Source: three-view drawing plus pictorial views. Frame: mm from the lowest corner of the part. A direction names the side the tool comes from. Give positions to 0.01 mm unless a question says otherwise; leave off trailing zeros. Order: outer loops, then holes, each group sorted by start corner. A loop starts at its lowest first (then second) coordinate and runs counter-clockwise, first axis right, second up. Notation, with made-up numbers: M -10,26.25 L 44,26.25 A17 ccw 44,42.25 Z; hole C 81.5,-26 d9. An arc over 180 degrees is marked long. One line per item, written item: value. Start each with the question number.
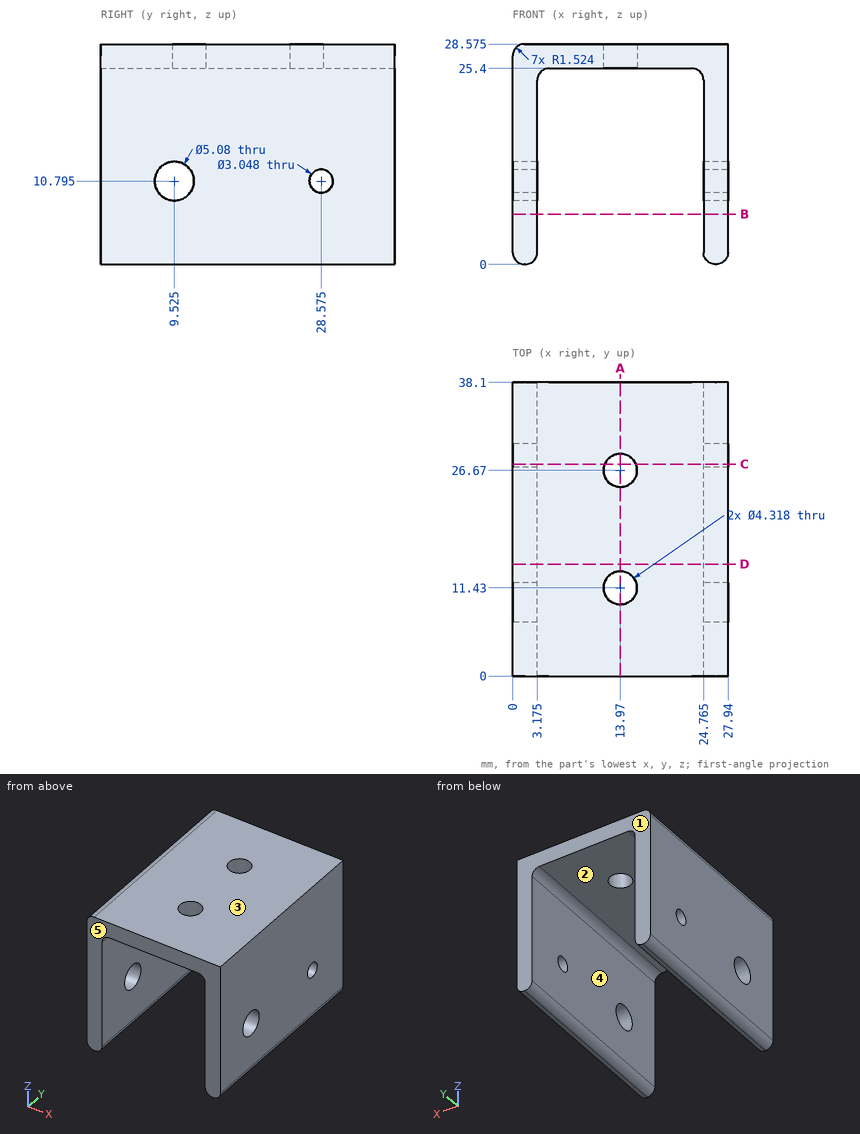
Q1. Mould query, pull axis Z, two halves, no side actions, for the marked faces 1, 2 and 3. Classes: +Z half, -Z half, draft (parallel to the pull), parting line (faces both ways), or undercut.
Q2. Section query A-A on x = 13.97. Return loops of the section in (y, z) (3 decimals), and give its area (3 significant figures).
Q3. Contact query for a flat-ended pin moving along its axis: pin 1 (3.5 mm diameter, centred on x = 13.97, y = 11.43, fed in from -Z). Output: stop coordinate, or through.
Q4. Section query B-B on z = 6.5. Return loops of the section in (x, y) (3 decimals).
Q5. Section query D-D on y = 14.5. Return loops of the section in (x, z) (3 decimals).
Q6. Section query C-C on y = 27.5. Return loops of the section in (x, z) (3 decimals), and give its area (3 significant figures).
Q7. Set-up query: the marked faces 4 and 5. Return all of +Z, -Z, +X, -X, +Y, -Y with unobstructed straight access to the full face (end or side cutting, diameter ignored); none if empty.
Q8. Ray query, line 1 along Y through (x, z) = (13.97, 27.5); line 2 along X through (y, z) = (23.5, 19.5) (3 decimals); line 3 along Y through (x, z) = (26, 9.5). Return the intervals inside material, ascending. Write a range as [from, to].
Results below:
1. face 1: draft
1. face 2: -Z half
1. face 3: +Z half
2. outline: M 0,25.4 L 9.271,25.4 L 9.271,28.575 L 0,28.575 Z; M 13.589,25.4 L 24.511,25.4 L 24.511,28.575 L 13.589,28.575 Z; M 28.829,25.4 L 38.1,25.4 L 38.1,28.575 L 28.829,28.575 Z
2. area: 93.5 mm2
3. pin 1: through
4. outline: M 0,0 L 3.175,0 L 3.175,38.1 L 0,38.1 Z; M 24.765,0 L 27.94,0 L 27.94,38.1 L 24.765,38.1 Z
5. outline: M 0,1.524 A1.524 ccw 1.524,0 L 1.651,0 A1.524 ccw 3.175,1.524 L 3.175,23.876 A1.524 cw 4.699,25.4 L 23.241,25.4 A1.524 cw 24.765,23.876 L 24.765,1.524 A1.524 ccw 26.289,0 L 26.416,0 A1.524 ccw 27.94,1.524 L 27.94,28.575 L 1.524,28.575 A1.524 ccw 0,27.051 Z
6. outline: M 0,1.524 A1.524 ccw 1.524,0 L 1.651,0 A1.524 ccw 3.175,1.524 L 3.175,9.715 L 0,9.715 Z; M 0,11.875 L 3.175,11.875 L 3.175,23.876 A1.524 cw 4.699,25.4 L 11.977,25.4 L 11.977,28.575 L 1.524,28.575 A1.524 ccw 0,27.051 Z; M 15.963,25.4 L 23.241,25.4 A1.524 cw 24.765,23.876 L 24.765,11.875 L 27.94,11.875 L 27.94,28.575 L 15.963,28.575 Z; M 24.765,1.524 A1.524 ccw 26.289,0 L 26.416,0 A1.524 ccw 27.94,1.524 L 27.94,9.715 L 24.765,9.715 Z
6. area: 222 mm2
7. face 4: -Z, +Y, -Y
7. face 5: +Z, -Z, +X, -X, -Y
8. line 1: [0, 9.27], [13.59, 24.51], [28.83, 38.1]
8. line 2: [0, 3.175], [24.765, 27.94]
8. line 3: [0, 7.34], [11.71, 27.77], [29.38, 38.1]
